Source: CAD feature listing. Evaluate the final solid. Frame: model axes, mm. A direction names the side the tool comes from. Give positions to 0.01 mm unless a question says otherwise; leave off trailing zeros. Loops run counter-clockwise (first coordinate to the right, second up) from the corner with the lowest first, then second, coordinate; pieces in that order, holes last. Notation, with made-up numbers: M 10.5,84.25 L 58.5,84.25 A8 cw 58.5,98.25 Z; hole C 18.5,77 d11. An arc over 180 degrees is marked long. Answer in a Markdown table with one row per item.
```python
from build123d import *

# Parameters (mm, degrees)
ESTRUSIONE_ESTRUSIONE1_DEPTH = 18
TAGLIO_ESTRUSIONE1_DEPTH     = 47
TAGLIO_ESTRUSIONE2_DEPTH     = 32
TAGLIO_ESTRUSIONE3_DEPTH     = 50
TAGLIO_ESTRUSIONE4_DEPTH     = 44
TAGLIO_ESTRUSIONE5_DEPTH     = 38
TAGLIO_ESTRUSIONE6_DEPTH     = 44


with BuildPart() as part:
    # Model → Estrusione-Estrusione1 (new body)
    with BuildSketch(Plane.XY):
        with BuildLine():
            Line((-275, -232), (-275, 232))
            Line((-275, 232), (-231.35, 232))
            ThreePointArc((-231.35, 232), (-228.175, 228.825), (-225, 232))
            Line((-225, 232), (-225, 250))
            Line((-225, 250), (-175, 250))
            Line((-175, 250), (-175, 232))
            ThreePointArc((-175, 232), (-171.825, 228.825), (-168.65, 232))
            Line((-168.65, 232), (-131.35, 232))
            ThreePointArc((-131.35, 232), (-128.175, 228.825), (-125, 232))
            Line((-125, 232), (-125, 250))
            Line((-125, 250), (-75, 250))
            Line((-75, 250), (-75, 232))
            ThreePointArc((-75, 232), (-71.825, 228.825), (-68.65, 232))
            Line((-68.65, 232), (-31.35, 232))
            ThreePointArc((-31.35, 232), (-28.175, 228.825), (-25, 232))
            Line((-25, 232), (-25, 250))
            Line((-25, 250), (25, 250))
            Line((25, 250), (25, 232))
            ThreePointArc((25, 232), (28.175, 228.825), (31.35, 232))
            Line((31.35, 232), (68.65, 232))
            ThreePointArc((68.65, 232), (71.825, 228.825), (75, 232))
            Line((75, 232), (75, 250))
            Line((75, 250), (125, 250))
            Line((125, 250), (125, 232))
            ThreePointArc((125, 232), (128.175, 228.825), (131.35, 232))
            Line((131.35, 232), (168.65, 232))
            ThreePointArc((168.65, 232), (171.825, 228.825), (175, 232))
            Line((175, 232), (175, 250))
            Line((175, 250), (225, 250))
            Line((225, 250), (225, 232))
            ThreePointArc((225, 232), (228.175, 228.825), (231.35, 232))
            Line((231.35, 232), (275, 232))
            Line((275, 232), (275, -232))
            Line((275, -232), (231.35, -232))
            ThreePointArc((231.35, -232), (228.175, -228.825), (225, -232))
            Line((225, -232), (225, -250))
            Line((225, -250), (175, -250))
            Line((175, -250), (175, -232))
            ThreePointArc((175, -232), (171.825, -228.825), (168.65, -232))
            Line((168.65, -232), (131.35, -232))
            ThreePointArc((131.35, -232), (128.175, -228.825), (125, -232))
            Line((125, -232), (125, -250))
            Line((125, -250), (75, -250))
            Line((75, -250), (75, -232))
            ThreePointArc((75, -232), (71.825, -228.825), (68.65, -232))
            Line((68.65, -232), (31.35, -232))
            ThreePointArc((31.35, -232), (28.175, -228.825), (25, -232))
            Line((25, -232), (25, -250))
            Line((25, -250), (-25, -250))
            Line((-25, -250), (-25, -232))
            ThreePointArc((-25, -232), (-28.175, -228.825), (-31.35, -232))
            Line((-31.35, -232), (-68.65, -232))
            ThreePointArc((-68.65, -232), (-71.825, -228.825), (-75, -232))
            Line((-75, -232), (-75, -250))
            Line((-75, -250), (-125, -250))
            Line((-125, -250), (-125, -232))
            ThreePointArc((-125, -232), (-128.175, -228.825), (-131.35, -232))
            Line((-131.35, -232), (-168.65, -232))
            ThreePointArc((-168.65, -232), (-171.825, -228.825), (-175, -232))
            Line((-175, -232), (-175, -250))
            Line((-175, -250), (-225, -250))
            Line((-225, -250), (-225, -232))
            ThreePointArc((-225, -232), (-228.175, -228.825), (-231.35, -232))
            Line((-231.35, -232), (-275, -232))
        make_face()
    extrude(amount=ESTRUSIONE_ESTRUSIONE1_DEPTH)

    # Model<3> → Taglio-Estrusione1 (cut)
    with BuildSketch(Plane.XY):
        with BuildLine():
            Line((-255, 145.65), (-255, 108.35))
            ThreePointArc((-255, 108.35), (-258.175, 105.175), (-255, 102))
            Line((-255, 102), (-237, 102))
            ThreePointArc((-237, 102), (-233.825, 105.175), (-237, 108.35))
            Line((-237, 108.35), (-237, 145.65))
            ThreePointArc((-237, 145.65), (-233.825, 148.825), (-237, 152))
            Line((-237, 152), (-255, 152))
            ThreePointArc((-255, 152), (-258.175, 148.825), (-255, 145.65))
        make_face()
    extrude(amount=TAGLIO_ESTRUSIONE1_DEPTH, mode=Mode.SUBTRACT)

    # Model<4> → Taglio-Estrusione2 (cut)
    with BuildSketch(Plane.XY):
        with BuildLine():
            Line((-255, -18.65), (-255, 18.65))
            ThreePointArc((-255, 18.65), (-258.175, 21.825), (-255, 25))
            Line((-255, 25), (-237, 25))
            ThreePointArc((-237, 25), (-233.825, 21.825), (-237, 18.65))
            Line((-237, 18.65), (-237, -18.65))
            ThreePointArc((-237, -18.65), (-233.825, -21.825), (-237, -25))
            Line((-237, -25), (-255, -25))
            ThreePointArc((-255, -25), (-258.175, -21.825), (-255, -18.65))
        make_face()
    extrude(amount=TAGLIO_ESTRUSIONE2_DEPTH, mode=Mode.SUBTRACT)

    # Model<5> → Taglio-Estrusione3 (cut)
    with BuildSketch(Plane.XY):
        with BuildLine():
            Line((-255, -145.65), (-255, -108.35))
            ThreePointArc((-255, -108.35), (-258.175, -105.175), (-255, -102))
            Line((-255, -102), (-237, -102))
            ThreePointArc((-237, -102), (-233.825, -105.175), (-237, -108.35))
            Line((-237, -108.35), (-237, -145.65))
            ThreePointArc((-237, -145.65), (-233.825, -148.825), (-237, -152))
            Line((-237, -152), (-255, -152))
            ThreePointArc((-255, -152), (-258.175, -148.825), (-255, -145.65))
        make_face()
    extrude(amount=TAGLIO_ESTRUSIONE3_DEPTH, mode=Mode.SUBTRACT)

    # Model<6> → Taglio-Estrusione4 (cut)
    with BuildSketch(Plane.XY):
        with BuildLine():
            Line((237, 145.65), (237, 108.35))
            ThreePointArc((237, 108.35), (233.825, 105.175), (237, 102))
            Line((237, 102), (255, 102))
            ThreePointArc((255, 102), (258.175, 105.175), (255, 108.35))
            Line((255, 108.35), (255, 145.65))
            ThreePointArc((255, 145.65), (258.175, 148.825), (255, 152))
            Line((255, 152), (237, 152))
            ThreePointArc((237, 152), (233.825, 148.825), (237, 145.65))
        make_face()
    extrude(amount=TAGLIO_ESTRUSIONE4_DEPTH, mode=Mode.SUBTRACT)

    # Model<7> → Taglio-Estrusione5 (cut)
    with BuildSketch(Plane.XY):
        with BuildLine():
            Line((237, -18.65), (237, 18.65))
            ThreePointArc((237, 18.65), (233.825, 21.825), (237, 25))
            Line((237, 25), (255, 25))
            ThreePointArc((255, 25), (258.175, 21.825), (255, 18.65))
            Line((255, 18.65), (255, -18.65))
            ThreePointArc((255, -18.65), (258.175, -21.825), (255, -25))
            Line((255, -25), (237, -25))
            ThreePointArc((237, -25), (233.825, -21.825), (237, -18.65))
        make_face()
    extrude(amount=TAGLIO_ESTRUSIONE5_DEPTH, mode=Mode.SUBTRACT)

    # Model<10> → Taglio-Estrusione6 (cut)
    with BuildSketch(Plane.XY):
        with BuildLine():
            Line((237, -145.65), (237, -108.35))
            ThreePointArc((237, -108.35), (233.825, -105.175), (237, -102))
            Line((237, -102), (255, -102))
            ThreePointArc((255, -102), (258.175, -105.175), (255, -108.35))
            Line((255, -108.35), (255, -145.65))
            ThreePointArc((255, -145.65), (258.175, -148.825), (255, -152))
            Line((255, -152), (237, -152))
            ThreePointArc((237, -152), (233.825, -148.825), (237, -145.65))
        make_face()
    extrude(amount=TAGLIO_ESTRUSIONE6_DEPTH, mode=Mode.SUBTRACT)


solid = part.part
```
1) Material intervals for L1, parallel to X at y = 113, z = 11.5; L2, parallel to Y at x = -25.5, z = 11.75, sorted ascending.
Reply:
| item | result |
|---|---|
| L1 | x = -275 to -255, -237 to 237, 255 to 275 |
| L2 | y = -230.29 to 230.29 |
2) Pin query (flat end, axial travel): pin 1 Ø3 at (x, z) = (30.5, 3) entering from +Y; pin 2 Ø5.5 at (x, z) = (152.5, 7) entering from -Y. Return the tip coordinate at first contact, or that it passes through.
Reply:
| item | result |
|---|---|
| pin 1 | stops at y = 232 |
| pin 2 | stops at y = -232 |
3) Section A-A, the plane x = -139. Return loops of the section in (y, z).
Reply:
| item | result |
|---|---|
| outline | M -232,0 L 232,0 L 232,18 L -232,18 Z |
4) Set-up query: faces 4 (the flat face through (-200, -250, 9)), 5 (the flat face through (-237, -127, 9)), 6 (the flat face through (-50, 232, 9)), 7 (the flat face through (0, 250, 9)), 8 (the flat face through (253, -232, 9)). Return all of +Z, -Z, +X, -X, +Y, -Y with unobstructed straight access to the full face (end or side cutting, diameter ignored); none if empty.
Reply:
| item | result |
|---|---|
| face 4 | +Z, -Z, +X, -X, -Y |
| face 5 | +Z, -Z |
| face 6 | +Z, -Z, +Y |
| face 7 | +Z, -Z, +X, -X, +Y |
| face 8 | +Z, -Z, +X, -Y |
5) Pull-direction query (Y, two-part tool) for faces 1 (the flat face through (-125, -241, 9)), 2 (the flat face through (100, -250, 9)), 3 (the flat face through (-255, 0, 9)); classes: released by +Y, released by -Y, zero draft, split by the parting line, or undercut.
Reply:
| item | result |
|---|---|
| face 1 | zero draft |
| face 2 | released by -Y |
| face 3 | undercut |
6) Section B-B, the plane z = 7. Count the separate pieces of the cut face and the enclosed holes in it, then the cut area to 3 significant figures.
Reply:
| item | result |
|---|---|
| separate pieces | 1 |
| enclosed holes | 6 |
| area | 258,000 mm² |
